Read the model definition and answer for the solid it produces. Units are mm, in the model's axes. A direction names the side the tool comes from. Coordinates: 2 decimals unless noted, no trailing zeros. Write each loop counter-clockwise with the first axis right and the second up, starting at its lowest first coordinate (ties: lowest second). Pieces come first, ordered by that corner, then holes.
Item 1: Section C-C (y = 14) is taken. Give the vertices of the cut face in (x, z).
Item 2: Section A-A (z = 3) is taken. Give the vertices of the cut face in (x, y).
Item 3: A tool of negligible diameter and unlimited length cuts with its end or side. For faces 4 (the face through (8.445, 9.741, -0.315)), 5 (the face through (24.132, 30.213, 0.315)), 6 (the face through (11, 32, 0)), from which of +Z, -Z, +X, -X, +Y, -Y can it reach the whole face along a straight path? Write none if from no direction.
Item 4: Section D-D (x = 39.5) is taken. Give the vertices of the cut face in (y, z).
Item 5: Straight lines are drawn through the part: probe 1 along Y at (x, z) = (13.5, -4); probe 2 along X at (y, z) = (11.5, 20); probe 3 along Y at (x, z) = (53.5, 16.5). For each, find the intervals that lie inside material, in ascending order.
Item 6: Each of these flat-tipped pins is pushed along its axis until it touches: P1, Ø8, axis at x = 28.5, z = 9.5, coming from the -Y side; P2, Ø3.5, axis at x = 10.5, z = -6, coming from the +Y side. Where does it stop, or does it pass through?
Item 7: Determine the mould class of faces 1 (the face through (22, 0, 0)), 2 (the face through (46.677, 30.632, 0.315)), 3 (the face through (84, 25, 0)) for opening direction X: released by +X, released by -X, zero draft, split by the parting line, or undercut.
Item 8: Section B-B (x = 9) is taken. Give the vertices of the cut face in (y, z).
from build123d import *

# Parameters (mm, degrees)
ESQUISSE2_R        = 7
BOSS_EXTRU_2_DEPTH = 22.5


with BuildPart() as part:
    # Esquisse2 → Boss.-Extru.2 (new body, symmetric)
    with BuildSketch(Plane.XY):
        with BuildLine():
            Line((48.833954843, -19), (55, -19))
            Line((55, -19), (84, 16))
            Line((84, 16), (84, 35))
            Line((84, 35), (79, 40))
            Line((79, 40), (55, 40))
            ThreePointArc((55, 40), (46.518108988, 30.544085173), (33.984940886, 28.476115714))
            Line((33.984940886, 28.476115714), (14, 32))
            Line((14, 32), (7, 32))
            Line((7, 32), (0, 25))
            Line((0, 25), (0, 7))
            Line((0, 7), (7, 0))
            Line((7, 0), (37.112513701, 0))
            ThreePointArc((37.112513701, 0), (40.377749482, -1.213413768), (42.058152443, -4.264705882))
            ThreePointArc((42.058152443, -4.264705882), (44.394982646, -12.115672061), (48.833954843, -19))
        make_face()
        with Locations((14, 14)):
            Circle(ESQUISSE2_R, mode=Mode.SUBTRACT)
    extrude(amount=BOSS_EXTRU_2_DEPTH, both=True)


solid = part.part
Established:
1. outline: (0, -22.5) - (7, -22.5) - (7, 22.5) - (0, 22.5) - close; (21, -22.5) - (82.34, -22.5) - (82.34, 22.5) - (21, 22.5) - close
2. outline: (0, 7) - (7, 0) - (37.11, 0) arc R5 cw to (42.06, -4.26) arc R29 ccw to (48.83, -19) - (55, -19) - (84, 16) - (84, 35) - (79, 40) - (55, 40) arc R19.15 cw to (33.98, 28.48) - (14, 32) - (7, 32) - (0, 25) - close; hole circle Ø14 at (14, 14)
3. face 4: +Z, -Z
3. face 5: +Z, -Z, +Y
3. face 6: +Z, -Z, -X, +Y
4. outline: (-0.61, -22.5) - (28.31, -22.5) - (28.31, 22.5) - (-0.61, 22.5) - close
5. probe 1: y = 0 to 7.02, 20.98 to 32
5. probe 2: x = 0 to 7.46, 20.54 to 80.27
5. probe 3: y = -19 to 37.11
6. P1: stops at y = 0
6. P2: stops at y = 32
7. face 1: zero draft
7. face 2: undercut
7. face 3: released by +X
8. outline: (0, -22.5) - (9.1, -22.5) - (9.1, 22.5) - (0, 22.5) - close; (18.9, -22.5) - (32, -22.5) - (32, 22.5) - (18.9, 22.5) - close
